CAD build for the part. Positions are in the model's coordinates, mm. Give positions to 0.01 mm unless a question says otherwise; leave off trailing zeros. Loops run counter-clockwise (first coordinate to the right, second up) from the corner with the lowest first, then second, coordinate; pieces in that order, holes last. Notation, with made-up numbers: M -16,55 L 16,55 A25 ccw 16,86 Z; hole C 10.5,65.5 d10. An arc over 180 degrees is marked long. One line per question, with ' | ' between items.
```python
from build123d import *

# Parameters (mm, degrees)
EXTRUDE_1_DEPTH       = 244
EXTRUDE_3_DEPTH       = 244
PATTERN_CURVE_1_COUNT = 11
PATTERN_CURVE_1_PITCH = 10
SKETCH_3_R            = 2.25
CUT_EXTRUDE_1_DEPTH   = 6
SKETCH_4_R            = 1.6
SKETCH_4_R_2          = 2.6
SKETCH_4_R_3          = 2.1
CUT_EXTRUDE_2_DEPTH   = 5.5


with BuildPart() as part:
    # Эскиз1 → Вытянуть1 (new body)
    with BuildSketch(Plane.XY):
        with BuildLine():
            Line((0, 40), (1.528979332, 40))
            ThreePointArc((1.528979332, 40), (2.225614441, 39.717425624), (2.528547087, 39.029399052))
            Line((2.528547087, 39.029399052), (3.5, 6))
            Line((3.5, 6), (118.5, 6))
            Line((118.5, 6), (119.471452913, 39.029399052))
            ThreePointArc((119.471452913, 39.029399052), (119.774385559, 39.717425624), (120.471020668, 40))
            Line((120.471020668, 40), (122, 40))
            Line((122, 40), (122, 0))
            Line((122, 0), (0, 0))
            Line((0, 0), (0, 40))
        make_face()
    extrude(amount=EXTRUDE_1_DEPTH)

    # Эскиз2 → Вытянуть3 (add)
    with BuildSketch(Plane.XY.offset(244)):
        with BuildLine():
            Line((10.5, 39.5), (9.25, 6))
            Line((9.25, 6), (12.75, 6))
            Line((12.75, 6), (11.5, 39.5))
            ThreePointArc((11.5, 39.5), (11, 40), (10.5, 39.5))
        make_face()
    extrude_3 = extrude(amount=-EXTRUDE_3_DEPTH)

    # Кривая1: Вытянуть3 ×11
    with Locations(*[(i * PATTERN_CURVE_1_PITCH, 0, 0) for i in range(1, PATTERN_CURVE_1_COUNT)]):
        add(extrude_3)

    # Эскиз3 → Вырез-Вытянуть1 (cut)
    with BuildSketch(Plane.XZ):
        with Locations((26, 236)):
            Circle(SKETCH_3_R)
        with Locations((96, 236)):
            Circle(SKETCH_3_R)
        with Locations(Location((96, 8, 0), (0, 0, 180))):
            Circle(SKETCH_3_R)
        with Locations(Location((26, 8, 0), (0, 0, 180))):
            Circle(SKETCH_3_R)
    extrude(amount=-CUT_EXTRUDE_1_DEPTH, mode=Mode.SUBTRACT)

    # Эскиз4 → Вырез-Вытянуть2 (cut)
    with BuildSketch(Plane(origin=(-5.723570629, 0, -26.359021189), x_dir=(1, 0, 0), z_dir=(0, -1, 0))):
        with Locations((55.723570629, 158.359021189)):
            Circle(SKETCH_4_R)
        with Locations((55.723570629, 53.359021189)):
            Circle(SKETCH_4_R)
        with Locations((55.723570629, 173.359021189)):
            Circle(SKETCH_4_R)
        with Locations((73.723570629, 86.359021189)):
            Circle(SKETCH_4_R)
        with Locations((73.723570629, 134.359021189)):
            Circle(SKETCH_4_R)
        with Locations((84.723570629, 110.359021189)):
            Circle(SKETCH_4_R_2)
        with Locations((17.723570629, 220.359021189)):
            Circle(SKETCH_4_R_3)
    extrude(amount=-CUT_EXTRUDE_2_DEPTH, mode=Mode.SUBTRACT)


solid = part.part
```
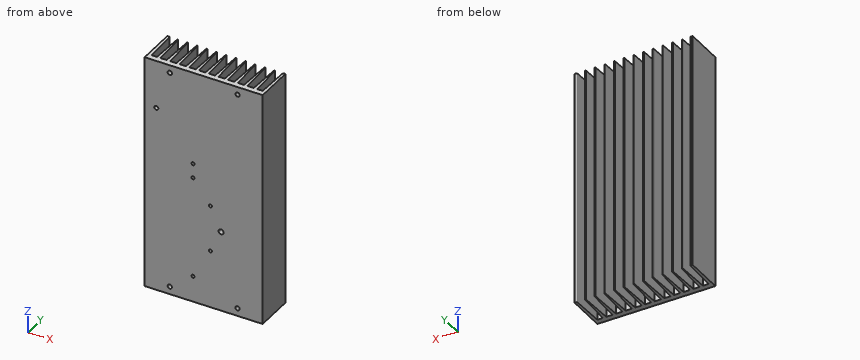
Item 1: Drill centre lines: line 1 along X through (y, z) = (3.65, 8); line 2 along Z through (x, y) = (50, 4.3); line 3 along Z through (x, y) = (26, 3). Where is each one in solid material? Low to high. Write a range as [from, to].
Conclusion:
line 1: [0, 23.75], [28.25, 93.75], [98.25, 122] | line 2: [0, 25.4], [28.6, 130.4], [133.6, 145.4], [148.6, 244] | line 3: [0, 5.75], [10.25, 233.75], [238.25, 244]
Item 2: Drop flat-ended pins along their axis: P1, Ø3, axis at x = 37, z = 160.5, coming from the +Y side; P2, Ø3, axis at x = 50, z = 147, coming from the -Y side; P3, Ø1.5, axis at x = 82, z = 94.5, coming from the +Y side. Give the stop position or say it passes through.
Conclusion:
P1: y = 6 | P2: y = 5.5 | P3: y = 39.93
Item 3: Saw through at B-B on x = 45.5. Give the cut face in (y, z), and give its area (3 significant figures).
Conclusion:
outline: M 0,0 L 6,0 L 6,244 L 0,244 Z | area: 1,460 mm²
Item 4: Saw through at A-A on y = 20. State how many separate pieces and enclosed holes the cut face has, and give its area (3 significant figures).
Conclusion:
separate pieces: 13 | enclosed holes: 0 | area: 8,100 mm²
